Build history of the part. All positions in model axes, mm. Face numbers are marked on the shaded views. A direction names the side the tool comes from. Coordinates: 2 decimals unless noted, no trailing zeros. Order: outer loops, then holes, each group sorted by start corner. A loop starts at its lowest first (then second) coordinate and runs counter-clockwise, first axis right, second up. Notation, with made-up numbers: M 37,-21.5 L 83,-21.5 A7 ccw 83,-12.5 Z; hole C 53.5,-15.5 d4. An arc over 180 degrees is marked long. Write item = value, one per line. Start each with the question number.
Q1. Drill centre lines: probe 1 along Z at (x, y) = (-25, 18.5) (3 decimals); probe 2 along X at (y, z) = (-14.5, 27) (3 decimals). Where is each one in solid material? Low to high.
Q2. Band-saw the part on A-A on z = 3.5. Write the cut outline in (x, y) (3 decimals).
Q3. Pin check, flat tips, straight feed: P1, Ø2, axis at x = -15.5, z = 29.5, coming from the -Y side (3 decimals); P2, Ø11, axis at y = 27, z = 15.5, coming from the +X side (3 decimals); P3, Ø1.5, axis at x = -16, z = 30.5, coming from the +Y side (3 decimals). Stop position of each tip, or through.
Q4. Band-saw the part on B-B on y = -40. Write the cut outline in (x, z) (3 decimals).
Q5. 3-axis set-ups, long thin cutter, end or side, ignore diameter. For the marked faces 1, 2 and 3: which of +Z, -Z, +X, -X, +Y, -Y reach the whole face in a straight line?
Q6. Band-saw the part on C-C on x = 100. Write the cut outline in (y, z) (3 decimals).
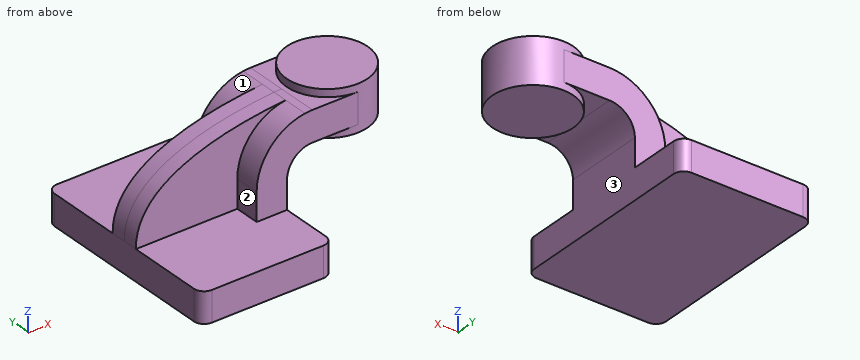
```python
from build123d import *

# Parameters (mm, degrees)
F1_DEPTH = 63.5
F2_DEPTH = 25.4
F0_W     = 25.4
F0_H     = 19.05
F3_DEPTH = 25.4
F4_DEPTH = 9.525
F6_R     = 6.35


with BuildPart() as f1:
    # F0 (on Front) → F1 (new body, symmetric)
    with BuildSketch(Plane.XZ):
        Polygon((-41.275, 9.525), (-41.275, -9.525), (41.275, -9.525), (41.275, 9.525), (22.225, 9.525), align=None)
    extrude(amount=F1_DEPTH, both=True)

    # F0 (on Front) → F2 (join, symmetric)
    with BuildSketch(Plane.XZ):
        with BuildLine():
            Line((22.225, 9.525), (41.275, 9.525))
            Line((41.275, 9.525), (41.275, 27.0002))
            ThreePointArc((41.275, 27.0002), (45.9246798487, 38.2255201513), (57.15, 42.8752))
            Line((57.15, 42.8752), (60.325, 42.8752))
            Line((60.325, 42.8752), (60.325, 61.9252))
            Line((60.325, 61.9252), (57.15, 61.9252))
            add(Edge.make_bspline(
                [(52.5691994145, 61.6234853871), (54.1342180077, 61.7382540245), (55.6631122744, 61.8383375559), (57.15, 61.9252)],
                knots=[106.979089872, 106.979089872, 106.979089872, 106.979089872, 111.5045361635, 111.5045361635, 111.5045361635, 111.5045361635], degree=3))
            ThreePointArc((52.5691994145, 61.6234853871), (30.8846227378, 50.0194437381), (22.225, 27.0002))
            Line((22.225, 27.0002), (22.225, 9.525))
        make_face()
    extrude(amount=F2_DEPTH, both=True)

    # F0 (on Front) → F3 (join, symmetric)
    with BuildSketch(Plane.XZ):
        with Locations((73.025, 52.4002)):
            Rectangle(F0_W, F0_H)
    extrude(amount=F3_DEPTH, both=True)

    # F0 (on Front) → F4 (join, symmetric)
    with BuildSketch(Plane.XZ):
        with BuildLine():
            add(Edge.make_bspline(
                [(-41.275, 9.525), (-41.6103147377, 47.9909608726), (15.5730107622, 58.9104171977), (52.5691994145, 61.6234853871)],
                knots=[0, 0, 0, 0, 106.979089872, 106.979089872, 106.979089872, 106.979089872], degree=3))
            Line((-41.275, 9.525), (22.225, 9.525))
            Line((22.225, 9.525), (22.225, 27.0002))
            ThreePointArc((22.225, 27.0002), (30.8846227378, 50.0194437381), (52.5691994145, 61.6234853871))
        make_face()
    extrude(amount=F4_DEPTH, both=True)

    # F0 (on Front) → F5 (revolve)
    with BuildSketch(Plane.XZ):
        Polygon((85.725, 66.675), (85.725, 61.9252), (85.725, 42.8752), (85.725, 38.1), (111.125, 38.1), (111.125, 66.675), align=None)
    revolve(axis=Axis((85.725, 0, 52.3875), (0, 0, 1)))

    # F6
    f6_edges = [f1.edges().sort_by_distance(p)[0] for p in [
        (-41.275, -63.5, 0),
        (41.275, -63.5, 0),
        (41.275, 63.5, 0),
        (-41.275, 63.5, 0),
    ]]
    fillet(f6_edges, radius=F6_R)


solid = f1.part
```
Recorded:
q1.probe_1 = -9.525 to 9.525
q1.probe_2 = 22.225 to 41.275
q2.outline = M -41.275,-57.15 A6.35 ccw -34.925,-63.5 L 34.925,-63.5 A6.35 ccw 41.275,-57.15 L 41.275,57.15 A6.35 ccw 34.925,63.5 L -34.925,63.5 A6.35 ccw -41.275,57.15 Z
q3.P1 = -9.525
q3.P2 = 41.275
q3.P3 = 9.525
q4.outline = M -41.275,-9.525 L 41.275,-9.525 L 41.275,9.525 L -41.275,9.525 Z
q5.face_1 = +Z, -X, +Y
q5.face_2 = +Z, -X, -Y
q5.face_3 = -Z, +X, +Y, -Y
q6.outline = M -21.009,38.1 L 21.009,38.1 L 21.009,66.675 L -21.009,66.675 Z
